```python
from build123d import *

# Parameters (mm, degrees)
CROQUIS1_W              = 40
CROQUIS1_H              = 40
SALIENTE_EXTRUIR1_DEPTH = 7
CROQUIS3_W              = 5.6
CROQUIS3_H              = 5.7
SALIENTE_EXTRUIR3_DEPTH = 40
CROQUIS19_W             = 8
CROQUIS19_H             = 40
CORTAR_EXTRUIR5_DEPTH   = 5.7
CROQUIS20_R             = 2.5
CORTAR_EXTRUIR6_DEPTH   = 7
CROQUIS21_W             = 7
CROQUIS21_H             = 72
SALIENTE_EXTRUIR4_DEPTH = 50
CROQUIS22_R             = 5
CORTAR_EXTRUIR7_DEPTH   = 7
REDONDEO1_R             = 30
REDONDEO2_R             = 30
CROQUIS28_R             = 4.25
CORTAR_EXTRUIR11_DEPTH  = 3
CROQUIS29_W             = 113.908789422
CROQUIS29_H             = 183.564538758
CORTAR_EXTRUIR12_DEPTH  = 23


# Some blends are built 0.0001 mm under size
with BuildPart() as part:
    # Croquis1 → Saliente-Extruir1 (new body)
    with BuildSketch(Plane(origin=(0, 0, 0), x_dir=(1, 0, 0), z_dir=(0, 1, 0))):
        Rectangle(CROQUIS1_W, CROQUIS1_H)
    extrude(amount=SALIENTE_EXTRUIR1_DEPTH)

    # Croquis3 → Saliente-Extruir3 (add)
    with BuildSketch(Plane.ZY.offset(20)):
        with Locations((10, 9.85)):
            Rectangle(CROQUIS3_W, CROQUIS3_H)
        with Locations((-10, 9.85)):
            Rectangle(CROQUIS3_W, CROQUIS3_H)
    extrude(amount=-SALIENTE_EXTRUIR3_DEPTH)

    # Croquis19 → Cortar-Extruir5 (cut)
    with BuildSketch(Plane(origin=(0, 12.7, 0), x_dir=(1, 0, 0), z_dir=(0, 1, 0))):
        with Locations((-16, 0)):
            Rectangle(CROQUIS19_W, CROQUIS19_H)
        with Locations((16, 0)):
            Rectangle(CROQUIS19_W, CROQUIS19_H)
    extrude(amount=-CORTAR_EXTRUIR5_DEPTH, mode=Mode.SUBTRACT)

    # Croquis20 → Cortar-Extruir6 (cut)
    with BuildSketch(Plane(origin=(0, 7, 0), x_dir=(1, 0, 0), z_dir=(0, 1, 0))):
        with Locations(Location((-15.5, 10, 0), (0, 0, 270))):
            Circle(CROQUIS20_R)
        with Locations(Location((15.5, 10, 0), (0, 0, 270))):
            Circle(CROQUIS20_R)
        with Locations(Location((15.5, -10, 0), (0, 0, 270))):
            Circle(CROQUIS20_R)
        with Locations(Location((-15.5, -10, 0), (0, 0, 270))):
            Circle(CROQUIS20_R)
    extrude(amount=-CORTAR_EXTRUIR6_DEPTH, mode=Mode.SUBTRACT)

    # Croquis21 → Saliente-Extruir4 (add)
    with BuildSketch(Plane.XZ):
        with Locations((-6.5, 14)):
            Rectangle(CROQUIS21_W, CROQUIS21_H)
    extrude(amount=SALIENTE_EXTRUIR4_DEPTH)

    # Croquis22 → Cortar-Extruir7 (cut)
    with BuildSketch(Plane(origin=(-3, 0, 0), x_dir=(0, 0, -1), z_dir=(1, 0, 0))):
        with Locations((0, -30)):
            Circle(CROQUIS22_R)
    extrude(amount=-CORTAR_EXTRUIR7_DEPTH, mode=Mode.SUBTRACT)

    # Redondeo1
    redondeo1_edges = [part.edges().sort_by_distance(p)[0] for p in [
        (-6.5, 0, 50),
    ]]
    fillet(redondeo1_edges, radius=REDONDEO1_R - 0.0001)  # a hair under: the kernel refuses the full size

    # Redondeo2
    # the kernel refuses this fillet: 30 mm, written as the material it takes off along each edge
    with BuildSketch(Plane(origin=(67.710766507, -50, 50), x_dir=(0, 1, 0), z_dir=(-1, 0, 0))) as redondeo2_piece_1:
        with BuildLine():
            CenterArc((30, 28.284306603), REDONDEO2_R, 180, 70.528981937)
            Line((0, 28.284306603), (-0.6, 28.284306603))
            Line((-0.6, 28.284306603), (-0.6, 0))
            Line((-0.6, 0), (0, -0.6))
            ThreePointArc((0, -0.6), (10.00005, -0.6), (19.800102, -0.565686132))
            Line((19.800102, -0.565686132), (20.0001, 0))
        make_face()
    extrude(amount=148.421533013, mode=Mode.SUBTRACT)

    # Croquis28 → Cortar-Extruir11 (cut)
    with BuildSketch(Plane.ZY.offset(10)):
        with Locations((30, -30)):
            Circle(CROQUIS28_R)
    extrude(amount=-CORTAR_EXTRUIR11_DEPTH, mode=Mode.SUBTRACT)

    # Croquis29 → Cortar-Extruir12 (cut)
    with BuildSketch(Plane(origin=(20, 0, 0), x_dir=(0, 0, -1), z_dir=(1, 0, 0))):
        with Locations((0, 4.197692072)):
            Rectangle(CROQUIS29_W, CROQUIS29_H)
    extrude(amount=-CORTAR_EXTRUIR12_DEPTH, mode=Mode.SUBTRACT)


solid = part.part
```
For this review, take the finished solid that the model builds, in its own axes (mm). A direction names the side the tool comes from. Round coordinates to 2 decimals unless told otherwise and drop trailing zeros. Order: outer loops, then holes, each group sorted by start corner. A loop starts at its lowest first (then second) coordinate and runs counter-clockwise, first axis right, second up.
Q1. Machinability: for faces 1 (the flat face through (-10, -25, 13)), 2 (the flat face through (-8, 10, -12.8)), 3 (the flat face through (-8, 10, -7.2)), 4 (the flat face through (-12, 3, 20)), which of the approach directions +Z, -Z, +X, -X, +Y, -Y give a long, thin tool a straight path to every point of the face, cutting with its end or side? Answer none if there is none.
Findings below:
face 1: +Z, -Z, -X, -Y
face 2: -Z, +X, -X, +Y
face 3: +X, -X, +Y
face 4: +Z, +X, -X, +Y
Q2. We need section B-B, the plane x = -15.5. Give the boundary of the cut face in (y, z).
Findings below:
outline: (0, -20) - (7, -20) - (7, -12.5) - (0, -12.5) - close; (0, -7.5) - (7, -7.5) - (7, 7.5) - (0, 7.5) - close; (0, 12.5) - (7, 12.5) - (7, 20) - (0, 20) - close
Q3. We need section A-A, the plane z = 4. Give the boundary of the cut face in (x, y), plus the area to 3 significant figures.
Findings below:
outline: (-20, 0) - (-10, 0) - (-10, -27) - (-3, -27) - (-3, 7) - (-20, 7) - close; (-10, -50) - (-3, -50) - (-3, -33) - (-10, -33) - close
area: 427 mm2
Q4. Insertion check: P1, Ø4, axis at y = -30.5, z = 28, coming from the -X side; P2, Ø8, axis at x = -15.5, z = 10, coming from the -Y side; P3, Ø1.7, axis at x = -9.5, y = 11, coming from the +Z side. Each pin has a flat end and moves straight along its axis. Give the tip position at first contact, or say it passes through.
Findings below:
P1: stops at x = -7
P2: stops at y = 0
P3: stops at z = 12.8
Q5. Mouldability with a two-part tool opening along Z and no side actions: class faces 5 (the flat face through (-8, 12.7, 10)), 6 (the cylindrical face through (-6.45, -34.88, 1.08)), 7 (the cylindrical face through (-6.451, -9.021, 41.445)) as pulls with the +Z half, pulls with the -Z half, needs draft (parallel to the pull), parting line crosses it, or undercut.
Findings below:
face 5: needs draft
face 6: undercut
face 7: pulls with the +Z half
Q6. Wall thickness on line 1 (X direction, y = 2, z = 10); line 2 (X direction, y = -12, z = 35); line 3 (Z direction, x = -4, y = 3.5): over which ranges is each line inside the solid? List them lowest first.
Findings below:
line 1: x = -20 to -18, -13 to -3
line 2: x = -10 to -3
line 3: z = -20 to 20
Q7. We need section C-C, the plane y = -31. Give the boundary of the cut face in (x, z), plus the area to 3 significant figures.
Findings below:
outline: (-10, -22) - (-3, -22) - (-3, -4.9) - (-10, -4.9) - close; (-10, 4.9) - (-3, 4.9) - (-3, 49.63) - (-10, 49.63) - (-10, 34.13) - (-7, 34.13) - (-7, 25.87) - (-10, 25.87) - close
area: 408 mm2
